For this review, take the finished solid that the model builds, in its own axes (mm). A direction names the side the tool comes from. Round coordinates to 2 decimals unless told otherwise and drop trailing zeros. Write each loop counter-clockwise with the first axis right and the second up, starting at its lowest first coordinate (ties: lowest second). Pieces come first, ordered by that corner, then holes.
from build123d import *

# Parameters (mm, degrees)
SKETCH_1_R             = 16
EXTRUDE_1_DEPTH        = 3
SKETCH_2_R             = 8
EXTRUDE_2_DEPTH        = 10
SKETCH_3_R             = 4
CUT_EXTRUDE_1_DEPTH    = 14
SKETCH_5_R             = 1.5
CUT_EXTRUDE_3_DEPTH    = 4
HOLE_WIZARD_M4_1_D     = 3.3
HOLE_WIZARD_M4_1_DEPTH = 3
HOLE_WIZARD_M4_2_D     = 3.3


with BuildPart() as part:
    # 草图1 → 凸台-拉伸1 (new body)
    with BuildSketch(Plane.XY):
        Circle(SKETCH_1_R)
    extrude(amount=EXTRUDE_1_DEPTH)

    # 草图2 → 凸台-拉伸2 (add)
    with BuildSketch(Plane.XY.offset(3)):
        Circle(SKETCH_2_R)
    extrude(amount=EXTRUDE_2_DEPTH)

    # 草图3 → 切除-拉伸1 (cut, through all)
    with BuildSketch(Plane.XY.offset(13)):
        Circle(SKETCH_3_R)
    extrude(amount=-CUT_EXTRUDE_1_DEPTH, mode=Mode.SUBTRACT)

    # 草图5 → 切除-拉伸3 (cut, through all)
    with BuildSketch(Plane.XY.offset(3)):
        with Locations((-8.485281374, -8.485281374)):
            Circle(SKETCH_5_R)
        with Locations((-8.485281374, 8.485281374)):
            Circle(SKETCH_5_R)
        with Locations((8.485281374, -8.485281374)):
            Circle(SKETCH_5_R)
        with Locations((8.485281374, 8.485281374)):
            Circle(SKETCH_5_R)
    extrude(amount=-CUT_EXTRUDE_3_DEPTH, mode=Mode.SUBTRACT)

    # M4 螺纹孔1
    with Locations(Plane(origin=(-8.485281374, 8.485281374, 3), x_dir=(1, 0, 0), z_dir=(0, 0, 1))):
        with Locations((0, 0), (16.970562748, 0), (16.970562748, -16.970562748), (0, -16.970562748)):
            Hole(HOLE_WIZARD_M4_1_D / 2, depth=HOLE_WIZARD_M4_1_DEPTH)

    # M4 螺纹孔2 (through all)
    with Locations(Plane(origin=(8, 0, 7.5), x_dir=(0, 1, 0), z_dir=(1, 0, 0))):
        with Locations((0, 0)):
            Hole(HOLE_WIZARD_M4_2_D / 2)


solid = part.part
(1) Mouldability with a two-part tool opening along X and no side actions: class faces 3 (the face through (9.7, 9.6, 1.5)), 4 (the face through (5.79, 1.65, 7.57)), 5 (the face through (-8.27, 10.12, 1.48)), 6 (the face through (-3.47, -15.62, 1.48)) as pulls with the +X half, pulls with the -X half, needs draft (parallel to the pull), parting line crosses it, or undercut.
Geometry check:
face 3: undercut
face 4: needs draft
face 5: undercut
face 6: parting line crosses it
(2) We need section D-D, the plane x = 4.5. Give the boundary of the cut face in (y, z), and give its area (3 significant figures).
Geometry check:
outline: (-15.35, 0) - (15.35, 0) - (15.35, 3) - (6.61, 3) - (6.61, 13) - (-6.61, 13) - (-6.61, 3) - (-15.35, 3) - close; hole circle Ø3.3 at (0, 7.5)
area: 216 mm2
(3) For pin 1 Ø4.5 at (y, z) = (0, 7.5) entering from -X; pin 2 Ø4.5 at (x, y) = (8.49, 8.49) entering from +Z; pin 3 Ø3 at (x, y) = (8.49, -8.49) entering from -Z; pin 4 Ø5 at (y, z) = (-10, 1.5) entering from -X, all flat-tipped, find the tip position at first contact; note any pin that passes through.
Geometry check:
pin 1: stops at x = -8
pin 2: stops at z = 3
pin 3: passes through
pin 4: stops at x = -14.13
(4) We need section C-C, the plane z = 7.5. Give the boundary of the cut face in (x, y).
Geometry check:
outline: (-7.83, -1.65) arc R8 ccw to (7.83, -1.65) - (3.64, -1.65) arc R4 cw to (-3.64, -1.65) - close; (-7.83, 1.65) - (-3.64, 1.65) arc R4 cw to (3.64, 1.65) - (7.83, 1.65) arc R8 ccw to start
(5) For faces 1 (the face through (-3.2, -2.4, 6.6)), 2 (the face through (7.39, -3.06, 7.93)), list the 3-axis set-ups (+Z, -Z, +X, -X, +Y, -Y) from which the entire face can be reached by the end or side of a thin tool; tool diameter is ignored.
Geometry check:
face 1: +Z, -Z
face 2: +Z
(6) We need section B-B, the plane y = 0. Give the boundary of the cut face in (x, z).
Geometry check:
outline: (-16, 0) - (-4, 0) - (-4, 5.85) - (-8, 5.85) - (-8, 3) - (-16, 3) - close; (-8, 9.15) - (-4, 9.15) - (-4, 13) - (-8, 13) - close; (4, 0) - (16, 0) - (16, 3) - (8, 3) - (8, 5.85) - (4, 5.85) - close; (4, 9.15) - (8, 9.15) - (8, 13) - (4, 13) - close
(7) For line 1 along X through (y, z) = (0, 9.75); line 2 along Z through (x, y) = (10.5, 1), list the stretches that pass through material, from the lowest coordinate up.
Geometry check:
line 1: x = -8 to -4, 4 to 8
line 2: z = 0 to 3
(8) We need section A-A, the plane x = 0. Give the boundary of the cut face in (y, z), and give its area (3 significant figures).
Geometry check:
outline: (-16, 0) - (-4, 0) - (-4, 13) - (-8, 13) - (-8, 3) - (-16, 3) - close; (4, 0) - (16, 0) - (16, 3) - (8, 3) - (8, 13) - (4, 13) - close
area: 152 mm2
